Autodesk Inventor part; units mm, degrees
ref_plane "YZ Plane" through (0, 0, 0) normal (1, 0, 0) x (0, 1, 0)
ref_plane "XZ Plane" through (0, 0, 0) normal (0, 1, 0) x (-1, 0, 0)
ref_plane "XY Plane" through (0, 0, 0) normal (0, 0, 1) x (1, 0, 0)
sketch "Skizze1" plane through (0, 0, 0) normal (1, 0, 0) x (0, 1, 0)
  circle A0 centre (-22.8, 48.5) radius 11 construction
  circle A1 centre (-4.5, 41.3809) radius 6.5 construction
  line L0 (-97.6965, 0) -> (58.2827, 0)
  circle A2 centre (14.5, 21.5) radius 21.5 construction
  line L1 (-28, 10) -> (0, 10)
  line L2 (0, 10) -> (0, 35.3809)
  line L3 (-7, 0) -> (-7, 21.5) construction
  circle A3 centre (-4.5, 41.3809) radius 6 construction
  circle A4 centre (-4.5, 41.3809) radius 5 construction
  line L4 (-56.6136, 29) -> (0, 29) construction
  arc A5 (-28, 16) -> (-28, 10) centre (-28, 13) ccw
  line L5 (-75.4137, 30) -> (0, 30) construction
  line L6 (-28, 16) -> (-20, 16)
  line L7 (-20, 16) -> (-20, 42)
  line L8 (-20, 42) -> (-29, 42)
  line L9 (-29, 42) -> (-29, 57)
  circle A6 centre (-28, 13) radius 2
  circle A7 centre (-4.5, 41.3809) radius 5.5
  circle A8 centre (-22.8, 48.5) radius 0.5
  circle A9 centre (-3, 23) radius 0.8
  line L10 (14.5, 21.5) -> (-7, 21.5) construction
  line L11 (-29, 57) -> (0, 57)
  line L12 (-4.5, 41.3809) -> (-28, 13) construction
  line L13 (14.5, 21.5) -> (14.5, 20.5) construction
  line L14 (14.5, 20.5) -> (-4.5, 41.3809) construction
  circle A10 centre (-22.8, 48.5) radius 5 construction
  circle A11 centre (-12.7907, 47.1492) radius 5.1 construction
  circle A12 centre (-12.7907, 47.1492) radius 5.6 construction
  circle A13 centre (-12.7907, 47.1492) radius 1
  line L15 (0, 35.3809) -> (2, 35.3809)
  line L16 (2, 35.3809) -> (2, 47.3809)
  line L17 (2, 47.3809) -> (0, 47.3809)
  line L18 (0, 47.3809) -> (0, 57)
  line L19 (1, 41.3809) -> (-10, 41.3809) construction
  point P0 (0, 0)
  dimension "d4" = 43
  dimension "d0" = 22
  dimension "d2" = 13
  dimension "d5" = 10
  dimension "d6" = 7
  dimension "d7" = 12
  dimension "d8" = 10
  dimension "d9" = 29
  dimension "d11" = 30
  dimension "d12" = 4
  dimension "d14" = 6
  dimension "d15" = 28
  dimension "d16" = 20
  dimension "d17" = 42
  dimension "d19" = 29
  dimension "d20" = 11
  dimension "d33" = 1
  dimension "d34" = 48.5
  dimension "d36" = 1.6
  dimension "d37" = 3
  dimension "d54" = 57
  dimension "d58" = 1
  dimension "d59" = 81.925
  dimension "d65" = 10
  dimension "d66" = 10.2
  dimension "d67" = 0.5
  dimension "d68" = 2
  dimension "d69" = 2
  dimension "d70" = 6
  dimension "d72" = 1.5
  dimension "d73" = 22.8
extrude "Extrusion1" add sketch "Skizze1" along normal mid plane 5 contours A5 L6 L7 L8 L9 L11 L18 L17 L16 L15 L2 L1 | A8
sketch "Skizze2" plane through (-2.5, -29, 57) normal (0, 0, 1) x (1, 0, 0)
  line L0 (0, 0) -> (5, 0)
  line L1 (5, 5) -> (5, 0)
  line L2 (0, 0) -> (0, 5)
  line L3 (2.5, 29) -> (2.5, 0) construction
  line L4 (0, 0) -> (5, 0) construction
  line L5 (0, 5) -> (5, 5)
  line L6 (0, 29) -> (5, 29)
  line L7 (0, 29) -> (5, 29)
  point P0 (2.5, 26)
  point P1 (2.5, 3)
  dimension "d25" = 23
  dimension "d74" = 3
hole "Bohrung1" at (0, -3, 57) at (0, -26, 57) direction (0, 0, -1) diameter 2.459 depth 7 tip angle 118
fillet "Rundung1" radius 10 1 edges at (0, -29, 42)
sketch "Skizze3" plane through (-2.5, 0, 0) normal (-1, 0, 0) x (0, 0, 1)
  circle A0 centre (23, -3) radius 0.8
  line L0 (29, -4) -> (17, -4) construction
  circle A1 centre (23, -3) radius 0.8 construction
  line L1 (23, -4) -> (23, -3) construction
  point P0 (0, 0)
  point P1 (55, -8)
  dimension "d38" = 12
  dimension "d39" = 1
  dimension "d40" = 32
  dimension "d41" = 5
hole "Bohrung2" at (-2.5, -4, 17) at (-2.5, -4, 29) at (-2.5, -8, 55) direction (1, 0, 0) diameter 1.567 end through all
fillet "Rundung2" radius 4 2 edges at (0, -20, 42) (0, -20, 16)
fillet "Rundung3" radius 2 1 edges at (0, 0, 10)
fillet "Rundung4" radius 2 4 edges at (0, 0, 47.3809) (0, 2, 47.3809) (0, 2, 35.3809) (0, 0, 35.3809)
properties part number "Dribbler Seite" material "Aluminium 6061"
Input: part model. Units: mm. Frame: model coordinates. A direction names the side the tool comes from. Coordinates: 2 decimals unless noted, no trailing zeros. Write each loop counter-clockwise with the first axis right and the second up, starting at its lowest first coordinate (ties: lowest second). Pieces come first, ordered by that corner, then holes.
1) Set-up query: faces 1 (the cylindrical face through (-0.035, -20.724, 41.169)), 2 (the flat face through (0, 0, 23)), 3 (the cylindrical face through (0.471, -27.136, 53.451)), 4 (the flat face through (0, 0, 53)). Return all of +Z, -Z, +X, -X, +Y, -Y with unobstructed straight access to the full face (end or side cutting, diameter ignored); none if empty.
2) Section C-C on y = -8. Output: boundary loops of the cut face in (x, z).
3) Pin query (flat end, axial travel): pin 1 Ø1 at (x, z) = (1, 21) entering from +Y; pin 2 Ø2 at (x, z) = (1, 44) entering from -Y; pin 3 Ø1.5 at (x, z) = (-0.5, 55.5) entering from -Y; pin 4 Ø9 at (y, z) = (-4.5, 41.38) entering from +X. Return the tip coordinate at first contact, or that it passes through.
4) Section B-B on z = 13. Output: boundary loops of the cut face in (x, y), and give its area (3 significant figures).
5) Section D-D on y = -13. Output: boundary loops of the cut face in (x, z), and give its area (3 significant figures).
6) Mould query, pull axis Y, two halves, no side actions, for faces 5 (the flat face through (0, -26, 16)), 6 (the cylindrical face through (0.035, 0.275, 34.394)), 7 (the cylindrical face through (-0.04, -27.19, 46.21)), 8 (the conical face through (0.009, -25.787, 49.39)). Classes: pulls with the +Y half, pulls with the -Y half, needs draft (parallel to the pull), parting line crosses it, or undercut.
7) Material intervals for line 1 along Y through (x, z) = (0, 53); line 2 along Y through (x, z) = (0.8, 55); line 3 along Z through (x, y) = (0.35, -4), sorted ascending.
8) Section A-A on z = 55. Output: boundary loops of the cut face in (x, y).
Check result:
1. face 1: +X, -X, -Y
1. face 2: -Z, +X, -X, +Y
1. face 3: +Z
1. face 4: +Z, +X, -X, +Y
2. outline: (-2.5, 10) - (2.5, 10) - (2.5, 37.14) - (-2.5, 37.14) - close; (-2.5, 45.62) - (2.5, 45.62) - (2.5, 54.22) - (-2.5, 54.22) - close; (-2.5, 55.78) - (2.5, 55.78) - (2.5, 57) - (-2.5, 57) - close
3. pin 1: stops at y = 0
3. pin 2: stops at y = -26.19
3. pin 3: stops at y = -29
3. pin 4: passes through
4. outline: (-2.5, -31) - (2.5, -31) - (2.5, -30) - (-2.5, -30) - close; (-2.5, -26) - (2.5, -26) - (2.5, 0) - (-2.5, 0) - close
4. area: 135 mm2
5. outline: (-2.5, 10) - (2.5, 10) - (2.5, 46.17) - (-2.5, 46.17) - close; (-2.5, 48.13) - (2.5, 48.13) - (2.5, 57) - (-2.5, 57) - close
5. area: 225 mm2
6. face 5: needs draft
6. face 6: pulls with the +Y half
6. face 7: pulls with the -Y half
6. face 8: undercut
7. line 1: y = -29 to -27.23, -24.77 to -4.23, -1.77 to 0
7. line 2: y = -29 to -26.93, -25.07 to -8.78, -7.22 to -3.93, -2.07 to 0
7. line 3: z = 10 to 16.22, 17.78 to 28.22, 29.78 to 35.9, 46.86 to 49.9
8. outline: (-2.5, -29) - (2.5, -29) - (2.5, -8.78) - (-2.5, -8.78) - close; (-2.5, -7.22) - (2.5, -7.22) - (2.5, 0) - (-2.5, 0) - close; hole circle Ø2.46 at (0, -26); hole circle Ø2.46 at (0, -3)
